```python
from build123d import *

# Parameters (mm, degrees)
BOSS_EXTRUDE1_DEPTH   = 15.24
CAVITY1_OUTLINE_R     = 4.445
CAVITY1_OUTLINE_R_2   = 1.143
CAVITY1_DEPTH         = 10.16
CAVITY1_START         = 10.16
CAVITY1_2_OUTLINE_R   = 1.143
CAVITY1_2_OUTLINE_R_2 = 7.239
CAVITY1_2_DEPTH       = 5.08
CAVITY1_3_OUTLINE_R   = 4.445
CAVITY1_3_DEPTH       = 3.048
CAVITY1_4_DEPTH       = 1.778
CAVITY1_START_2       = 12.192
CAVITY1_5_OUTLINE_R   = 1.905
CAVITY1_5_OUTLINE_R_2 = 1.143
CAVITY1_5_DEPTH       = 3.048
CAVITY1_6_OUTLINE_R   = 2.286
CAVITY1_6_DEPTH       = 1.27
CAVITY1_START_3       = 13.208
CAVITY1_7_DEPTH       = 0.254
FILLET1_R             = 12.7
SKETCH2_R             = 2.286
CUT_EXTRUDE1_DEPTH    = 108.072373654
CUT_EXTRUDE2_DEPTH    = 50.8
CUT_EXTRUDE4_DEPTH    = 25.4
FILLET2_R             = 1.27


# Read off the part's stored shape, not the designer's step: Cavity1
with BuildPart() as part:
    # Sketch1 → Boss-Extrude1 (new body)
    with BuildSketch(Plane(origin=(0, 0, 0), x_dir=(1, 0, 0), z_dir=(0, 1, 0))):
        with BuildLine():
            Line((0, 0), (0, 76.2))
            Line((0, 76.2), (-73.66, 76.2))
            ThreePointArc((-73.66, 76.2), (-48.155396991, 41.704814738), (-38.1, 0))
            Line((-38.1, 0), (0, 0))
        make_face()
    extrude(amount=BOSS_EXTRUDE1_DEPTH)

    # Cavity1 outline → Cavity1 (cut)
    with BuildSketch(Plane(origin=(0, 0, 0), x_dir=(1, 0, 0), z_dir=(0, 1, 0))):
        with BuildLine():
            ThreePointArc((-11.560994253, 41.539188518), (-18.2245, 43.18), (-24.888005747, 41.539188518))
            ThreePointArc((-24.888005747, 41.539188518), (-28.461347552, 42.868105214), (-28.288628852, 39.059567504))
            ThreePointArc((-28.288628852, 39.059567504), (-32.5755, 28.829), (-28.288628852, 18.598432496))
            ThreePointArc((-28.288628852, 18.598432496), (-28.461347552, 14.789894786), (-24.888005747, 16.118811482))
            ThreePointArc((-24.888005747, 16.118811482), (-18.2245, 14.478), (-11.560994253, 16.118811482))
            ThreePointArc((-11.560994253, 16.118811482), (-7.987652448, 14.789894786), (-8.160371148, 18.598432496))
            ThreePointArc((-8.160371148, 18.598432496), (-3.8735, 28.829), (-8.160371148, 39.059567504))
            ThreePointArc((-8.160371148, 39.059567504), (-7.987652448, 42.868105214), (-11.560994253, 41.539188518))
        make_face()
        with Locations((-18.2245, 54.229)):
            Circle(CAVITY1_OUTLINE_R)
        with Locations((-4.2545, 63.373)):
            Circle(CAVITY1_OUTLINE_R_2)
        with Locations((-32.1945, 63.373)):
            Circle(CAVITY1_OUTLINE_R_2)
        with Locations((-4.2545, 19.685)):
            Circle(CAVITY1_OUTLINE_R_2)
        with Locations((-32.1945, 19.685)):
            Circle(CAVITY1_OUTLINE_R_2)
    extrude(amount=CAVITY1_DEPTH, mode=Mode.SUBTRACT)

    # Cavity1 2 outline → Cavity1 2 (cut)
    with BuildSketch(Plane(origin=(0, 0, 0), x_dir=(1, 0, 0), z_dir=(0, 1, 0)).offset(CAVITY1_START)):
        with Locations((-4.2545, 63.373)):
            Circle(CAVITY1_2_OUTLINE_R)
        with Locations((-32.1945, 63.373)):
            Circle(CAVITY1_2_OUTLINE_R)
        with Locations((-4.2545, 19.685)):
            Circle(CAVITY1_2_OUTLINE_R)
        with Locations((-32.1945, 19.685)):
            Circle(CAVITY1_2_OUTLINE_R)
        with Locations((-18.2245, 28.829)):
            Circle(CAVITY1_2_OUTLINE_R_2)
    extrude(amount=CAVITY1_2_DEPTH, mode=Mode.SUBTRACT)

    # Cavity1 3 outline → Cavity1 3 (cut)
    with BuildSketch(Plane(origin=(0, 0, 0), x_dir=(1, 0, 0), z_dir=(0, 1, 0)).offset(CAVITY1_START)):
        with BuildLine():
            ThreePointArc((-21.84493784, 42.715815), (-18.2245, 37.719), (-14.60406216, 42.715815))
            ThreePointArc((-14.60406216, 42.715815), (-18.2245, 43.18), (-21.84493784, 42.715815))
        make_face()
        with Locations((-18.2245, 54.229)):
            Circle(CAVITY1_3_OUTLINE_R)
    extrude(amount=CAVITY1_3_DEPTH, mode=Mode.SUBTRACT)

    # Cavity1 4 outline → Cavity1 4 (cut)
    with BuildSketch(Plane(origin=(0, 0, 0), x_dir=(1, 0, 0), z_dir=(0, 1, 0))):
        with BuildLine():
            Line((-16.979413564, 49.961941907), (-16.962599029, 49.910648336))
            ThreePointArc((-16.962599029, 49.910648336), (-13.643456381, 51.73666679), (-11.954738237, 55.127725966))
            Line((-11.954738237, 55.127725966), (-13.895987251, 53.218058667))
            ThreePointArc((-13.895987251, 53.218058667), (-14.996989185, 51.172662495), (-16.979413564, 49.961941907))
        make_face()
        with BuildLine():
            ThreePointArc((-17.321192174, 49.848577582), (-17.141450842, 49.87704351), (-16.962599029, 49.910648336))
            Line((-16.962599029, 49.910648336), (-16.979413564, 49.961941907))
            ThreePointArc((-16.979413564, 49.961941907), (-17.131364048, 49.920510846), (-17.284686925, 49.884488936))
            Line((-17.284686925, 49.884488936), (-17.321192174, 49.848577582))
        make_face()
        with BuildLine():
            Line((-19.469586436, 49.961941907), (-19.486400971, 49.910648336))
            ThreePointArc((-19.486400971, 49.910648336), (-19.307549158, 49.87704351), (-19.127807826, 49.848577582))
            Line((-19.127807826, 49.848577582), (-19.164313075, 49.884488936))
            ThreePointArc((-19.164313075, 49.884488936), (-19.317635952, 49.920510846), (-19.469586436, 49.961941907))
        make_face()
        with BuildLine():
            ThreePointArc((-24.494261763, 55.127725966), (-22.805543619, 51.73666679), (-19.486400971, 49.910648336))
            Line((-19.486400971, 49.910648336), (-19.469586436, 49.961941907))
            ThreePointArc((-19.469586436, 49.961941907), (-21.452010815, 51.172662495), (-22.553012749, 53.218058667))
            Line((-22.553012749, 53.218058667), (-24.494261763, 55.127725966))
        make_face()
        with BuildLine():
            ThreePointArc((-18.2245, 49.784), (-17.771693393, 49.800164971), (-17.321192174, 49.848577582))
            Line((-17.321192174, 49.848577582), (-17.284686925, 49.884488936))
            ThreePointArc((-17.284686925, 49.884488936), (-17.751914917, 49.809193631), (-18.2245, 49.784))
        make_face()
        with BuildLine():
            Line((-13.895987251, 53.218058667), (-11.954738237, 55.127725966))
            ThreePointArc((-11.954738237, 55.127725966), (-11.894591344, 55.629266009), (-11.8745, 56.134))
            ThreePointArc((-11.8745, 56.134), (-12.87382539, 59.553470897), (-15.557265738, 61.896669641))
            Line((-15.557265738, 61.896669641), (-16.701846661, 58.405068942))
            ThreePointArc((-16.701846661, 58.405068942), (-14.582644766, 56.7775124), (-13.7795, 54.229))
            ThreePointArc((-13.7795, 54.229), (-13.80871784, 53.720184793), (-13.895987251, 53.218058667))
        make_face()
        with BuildLine():
            Line((-19.164313075, 49.884488936), (-19.127807826, 49.848577582))
            ThreePointArc((-19.127807826, 49.848577582), (-18.677306607, 49.800164971), (-18.2245, 49.784))
            ThreePointArc((-18.2245, 49.784), (-18.697085083, 49.809193631), (-19.164313075, 49.884488936))
        make_face()
        with BuildLine():
            ThreePointArc((-20.891734262, 61.896669641), (-23.830044051, 59.117349777), (-24.494261763, 55.127725966))
            Line((-24.494261763, 55.127725966), (-22.553012749, 53.218058667))
            ThreePointArc((-22.553012749, 53.218058667), (-22.134142573, 56.3438806), (-19.747153339, 58.405068942))
            Line((-19.747153339, 58.405068942), (-20.891734262, 61.896669641))
        make_face()
        with BuildLine():
            ThreePointArc((-15.557265738, 61.896669641), (-18.2245, 62.484), (-20.891734262, 61.896669641))
            Line((-20.891734262, 61.896669641), (-19.747153339, 58.405068942))
            ThreePointArc((-19.747153339, 58.405068942), (-18.2245, 58.674), (-16.701846661, 58.405068942))
            Line((-16.701846661, 58.405068942), (-15.557265738, 61.896669641))
        make_face()
    extrude(amount=CAVITY1_4_DEPTH, mode=Mode.SUBTRACT)

    # Cavity1 5 outline → Cavity1 5 (cut)
    # profile 1 of 4: a face of its own
    with BuildSketch(Plane(origin=(0, 0, 0), x_dir=(1, 0, 0), z_dir=(0, 1, 0)).offset(CAVITY1_START_2)):
        with Locations((-4.2545, 63.373)):
            Circle(CAVITY1_5_OUTLINE_R)
        with Locations((-4.2545, 63.373)):
            Circle(CAVITY1_5_OUTLINE_R_2, mode=Mode.SUBTRACT)
    # profile 2 of 4: a face of its own
    with BuildSketch(Plane(origin=(0, 0, 0), x_dir=(1, 0, 0), z_dir=(0, 1, 0)).offset(CAVITY1_START_2)):
        with Locations((-32.1945, 63.373)):
            Circle(CAVITY1_5_OUTLINE_R)
        with Locations((-32.1945, 63.373)):
            Circle(CAVITY1_5_OUTLINE_R_2, mode=Mode.SUBTRACT)
    # profile 3 of 4: a face of its own
    with BuildSketch(Plane(origin=(0, 0, 0), x_dir=(1, 0, 0), z_dir=(0, 1, 0)).offset(CAVITY1_START_2)):
        with Locations((-4.2545, 19.685)):
            Circle(CAVITY1_5_OUTLINE_R)
        with Locations((-4.2545, 19.685)):
            Circle(CAVITY1_5_OUTLINE_R_2, mode=Mode.SUBTRACT)
    # profile 4 of 4: a face of its own
    with BuildSketch(Plane(origin=(0, 0, 0), x_dir=(1, 0, 0), z_dir=(0, 1, 0)).offset(CAVITY1_START_2)):
        with Locations((-32.1945, 19.685)):
            Circle(CAVITY1_5_OUTLINE_R)
        with Locations((-32.1945, 19.685)):
            Circle(CAVITY1_5_OUTLINE_R_2, mode=Mode.SUBTRACT)
    extrude(amount=CAVITY1_5_DEPTH, mode=Mode.SUBTRACT)

    # Cavity1 6 outline → Cavity1 6 (cut)
    with BuildSketch(Plane(origin=(0, 0, 0), x_dir=(1, 0, 0), z_dir=(0, 1, 0)).offset(CAVITY1_START)):
        with Locations((-9.3345, 41.021)):
            Circle(CAVITY1_6_OUTLINE_R)
        with Locations((-27.1145, 41.021)):
            Circle(CAVITY1_6_OUTLINE_R)
        with Locations((-9.3345, 16.637)):
            Circle(CAVITY1_6_OUTLINE_R)
        with Locations((-27.1145, 16.637)):
            Circle(CAVITY1_6_OUTLINE_R)
    extrude(amount=CAVITY1_6_DEPTH, mode=Mode.SUBTRACT)

    # Cavity1 7 outline → Cavity1 7 (cut)
    with BuildSketch(Plane(origin=(0, 0, 0), x_dir=(1, 0, 0), z_dir=(0, 1, 0)).offset(CAVITY1_START_3)):
        with BuildLine():
            ThreePointArc((-21.84493784, 42.715815), (-18.2245, 37.719), (-14.60406216, 42.715815))
            ThreePointArc((-14.60406216, 42.715815), (-18.2245, 43.18), (-21.84493784, 42.715815))
        make_face()
    extrude(amount=CAVITY1_7_DEPTH, mode=Mode.SUBTRACT)

    # Fillet1
    fillet1_edges = [part.edges().sort_by_distance(p)[0] for p in [
        (-38.1, 7.62, 0),
    ]]
    fillet(fillet1_edges, radius=FILLET1_R)

    # Sketch2 → Cut-Extrude1 (cut, through all)
    with BuildSketch(Plane(origin=(0, 0, 0), x_dir=(0, 0, -1), z_dir=(1, 0, 0))):
        with Locations((6.35, 7.62)):
            Circle(SKETCH2_R)
        with Locations((69.85, 7.62)):
            Circle(SKETCH2_R)
    extrude(amount=-CUT_EXTRUDE1_DEPTH, mode=Mode.SUBTRACT)

    # Sketch4 → Cut-Extrude2 (cut)
    with BuildSketch(Plane(origin=(-76.2, 0, 0), x_dir=(0, 0, -1), z_dir=(1, 0, 0))):
        Polygon((6.35, 2.286), (10.969379504, 4.953), (10.969379504, 10.287), (6.35, 12.954), (1.730620496, 10.287), (1.730620496, 4.953), align=None)
    extrude(amount=CUT_EXTRUDE2_DEPTH, mode=Mode.SUBTRACT)

    # Sketch4<4> → Cut-Extrude4 (cut)
    with BuildSketch(Plane(origin=(-76.2, 0, 0), x_dir=(0, 0, -1), z_dir=(1, 0, 0))):
        Polygon((69.85, 2.286), (74.469379504, 4.953), (74.469379504, 10.287), (69.85, 12.954), (65.230620496, 10.287), (65.230620496, 4.953), align=None)
    extrude(amount=CUT_EXTRUDE4_DEPTH, mode=Mode.SUBTRACT)

    # Fillet2
    # the kernel refuses this fillet: 1.27 mm, written as the material it takes off along each edge
    with BuildSketch(Plane(origin=(-73.66, -8.077592452, -76.2), x_dir=(0.7323839064135403, 0, 0.6808919250706698), z_dir=(0, 1, 0))) as fillet2_piece_1:
        with BuildLine():
            CenterArc((3.231092231, 1.269859429), FILLET2_R, 132.913380591, 136.234131595)
            Line((2.366359486, 2.19998699), (0, 0))
            ThreePointArc((0, 0), (1.606098477, 0.011948565), (3.212196954, 0))
        make_face()
    extrude(amount=31.395184904, mode=Mode.SUBTRACT)
    with BuildSketch(Plane(origin=(0, -3.175, 0), x_dir=(-1, 0, 0), z_dir=(0, 1, 0))) as fillet2_piece_2:
        with BuildLine():
            CenterArc((FILLET2_R, -FILLET2_R), FILLET2_R, 90, 90)
            Line((0, -FILLET2_R), (0, 0))
            Line((0, 0), (FILLET2_R, 0))
        make_face()
    extrude(amount=21.59, mode=Mode.SUBTRACT)
    with BuildSketch(Plane(origin=(0, -3.175, -76.2), x_dir=(-1, 0, 0), z_dir=(0, 1, 0))) as fillet2_piece_3:
        with BuildLine():
            CenterArc((FILLET2_R, FILLET2_R), FILLET2_R, 180, 90)
            Line((0, FILLET2_R), (0, 0))
            Line((0, 0), (FILLET2_R, 0))
        make_face()
    extrude(amount=21.59, mode=Mode.SUBTRACT)


solid = part.part
```
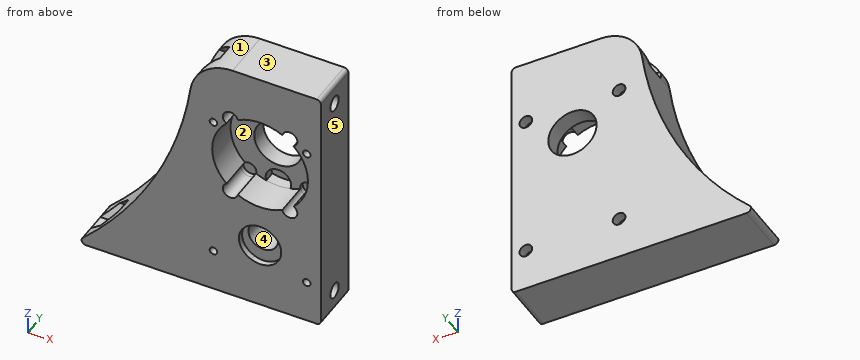
The model under review builds one solid part; all positions refer to its coordinate system, in mm. Face numbers are marked on the shaded views. A direction names the side the tool comes from. Round coordinates to 2 decimals unless told otherwise and drop trailing zeros. Loops run counter-clockwise (first coordinate to the right, second up) from the corner with the lowest first, then second, coordinate; pieces in that order, holes last. Notation, with made-up numbers: (87.25, 28) - (133.25, 28) arc R30 cw to (133.25, 61) - close; hole circle Ø8 at (48, 36.5). An arc over 180 degrees is marked (long way). Use a Markdown table: item, result. Add a question column.
Q1. Add section A-A (y = 7.62). State how many separate pieces and enclosed holes the cut face has, plus the area to 3 significant figures.
Q2. Machinability: for the marked faces 1 and 2, which of the approach directions +Z, -Z, +X, -X, +Y, -Y give a long, thin tool a straight path to every point of the face, cutting with its end or side? Answer none if there is none.
Q3. Insertion check: pin 1 Ø6 at (x, y) = (-34, 4.5) entering from +Z; pin 2 Ø1 at (x, z) = (-62, -61.5) entering from -Y; pin 3 Ø5 at (x, y) = (-60, 6) entering from +Z; pin 4 Ø2.5 at (x, z) = (-27.11, -16.64) entering from -Y. Each pin has a flat end and moves straight along its axis. Give the tip position at first contact, or say it passes through.
Q4. For probe 1 along Y at (x, z) = (-26.5, -69.85); probe 2 along X at (y, z) = (11.5, -62.5); probe 3 along X at (y, z) = (2.75, -19.5), list the stretches that pass through material, from the lowest coordinate up.
Q5. Add section D-D (z = -46). State the section outline as (x, y) points.
Q6. Add section C-C (x = -41.5). State the section outline as (y, z) points, plus the area to 3 significant figures.
Q7. Add section B-B (z = -23). State the section outline as (x, y) points, plus the area to 3 significant figures.
Q8. The part is to be moulded in two halves that separate along Z. For the marked faces 3, 4 and 5, say which applies: pulls with the +Z half, pulls with the -Z half, needs draft (parallel to the pull), parting line crosses it, or undercut.
Worked answers:
| question | item | result |
|---|---|---|
| 1 | separate pieces | 3 |
| 1 | enclosed holes | 6 |
| 1 | area | 2,370 mm² |
| 2 | face 1 | +Z, -X, +Y, -Y |
| 2 | face 2 | -Y |
| 3 | pin 1 | z = -0.83 |
| 3 | pin 2 | through |
| 3 | pin 3 | z = -57.9 |
| 3 | pin 4 | y = 11.43 |
| 4 | probe 1 | 0 to 5.33, 9.91 to 15.24 |
| 4 | probe 2 | -60.9 to -32.93, -31.46 to -4.99, -3.52 to 0 |
| 4 | probe 3 | -40.6 to -33.32, -31.07 to -29.13, -7.32 to -5.38, -3.13 to 0 |
| 5 | outline | (-50.28, 0) - (0, 0) - (0, 15.24) - (-50.28, 15.24) - close |
| 6 | outline | (0, -76.2) - (15.24, -76.2) - (15.24, -23.21) - (0, -23.21) - close; hole circle Ø4.57 at (7.62, -69.85) |
| 6 | area | 791 mm² |
| 7 | outline | (-41.44, 0) - (-31.34, 0) - (-31.34, 10.16) - (-22.52, 10.16) - (-22.52, 15.24) - (-41.44, 15.24) - close; (-13.93, 10.16) - (-5.11, 10.16) - (-5.11, 0) - (0, 0) - (0, 15.24) - (-13.93, 15.24) - close |
| 7 | area | 322 mm² |
| 8 | face 3 | pulls with the +Z half |
| 8 | face 4 | undercut |
| 8 | face 5 | needs draft |
